Can you work these out from the model? Positions are in its coordinate system, mm. A direction names the side the tool comes from. Coordinates: 2 decimals unless noted, no trailing zeros. Order: outer loops, then holes, each group sorted by start corner. A loop starts at its lowest first (then second) coordinate and runs counter-clockwise, first axis right, second up. Notation, with made-up numbers: (87, 5) -> (140, 5) arc R31 ccw to (140, 31) -> close; hole circle Ø6 at (0.5, 41.25). An arc over 180 degrees is marked (long way). Return JSON: item names as keys, results as strings. Group by question number.
1) Thinking about a two-plate mould opening in Z: for faces 1 (the flat face through (-3, 9, 292.1)), 2 (the flat face through (3, 9, -292.1)), 3 (the flat face through (134, 9, 209.55)), which applies, +Z half, -Z half, draft (parallel to the pull), parting line (faces both ways), or undercut?
2) If we section it at B-B, the plane y = 14: Please give me the cut outline in (x, z), then the cut area to 3 significant figures.
3) For faces 4 (the flat face through (209.55, 9, -112)), 5 (the flat face through (132, 9, 63.5)), 6 (the flat face through (-57.15, 9, 136)), which set-ups out of +Z, -Z, +X, -X, +Y, -Y let a thin tool reach every point of the face, with its end or its side?
4) If I drill on probe 1 along Z at (x, y) = (-160, 1.5); probe 2 along X at (y, z) = (12.25, 132), over which ranges is the centre line in solid material (lowest first)? Write a range as from..to.
5) If we section it at A-A, the plane x = 121: Please give me the cut outline in (y, z).
6) For pin 1 (5.5 mm diameter, centred on y = 9.5, z = 140.5, fed in from -X), with a flat end and sliding along its axis, tell me the tip position at first contact or that it passes through.
Autodesk Inventor part; units mm, degrees
ref_plane "XZ Plane" through (0, 0, 0) normal (0, 1, 0) x (-1, 0, 0)
ref_plane "XY Plane" through (0, 0, 0) normal (0, 0, 1) x (1, 0, 0)
sketch "Sketch1" plane through (0, 0, 0) normal (0, 1, 0) x (-1, 0, 0)
  line L0 (-209.55, 292.1) -> (-209.55, -292.1)
  line L1 (-209.55, -292.1) -> (209.55, -292.1)
  line L2 (209.55, -292.1) -> (209.55, 292.1)
  line L3 (209.55, 292.1) -> (-209.55, 292.1)
  line L4 (-209.55, 292.1) -> (209.55, -292.1) construction
  line L5 (-209.55, -292.1) -> (209.55, 292.1) construction
  point P0 (0, 0)
  dimension "baseLength" = 584.2
  dimension "baseWidth" = 419.1
extrude "Extrusion1" add sketch "Sketch1" along normal blind 17.78
sketch "Sketch2" plane through (0, 0, 0) normal (0, -1, 0) x (1, 0, 0)
  line L0 (209.55, 292.1) -> (209.55, -292.1)
  line L1 (209.55, 209.55) -> (57.15, 209.55)
  line L2 (57.15, 209.55) -> (57.15, 63.5)
  line L3 (57.15, 63.5) -> (209.55, 63.5)
  line L4 (209.55, 63.5) -> (209.55, 209.55)
  line L5 (-209.55, 292.1) -> (209.55, 292.1)
  point P0 (0, 0)
  dimension "backToEndOfGearBox" = 82.55
  dimension "backToFrontOfGearBox" = 228.6
  dimension "wdithForGearBox" = 152.4
extrude "Extrusion2" cut sketch "Sketch2" against normal through all
mirror "Mirror1" about plane through (0, 0, 0) normal (1, 0, 0) of "Extrusion2"
equation "\"baseLength\" = userBaseLength"
equation "\"baseWidth\" = userBaseWidth"
equation "\"spaceingAlongSides\" = 3.175"
equation "\"distanceFromBackForEndBolt\" = 38.1"
equation "\"spacingForBolt\" = 25.4"
equation "\"widthOfSpacingForBolt\" = 12.7"
equation "\"lengthOfSpacingForBolt\" = 25.4"
equation "\"userBaseWidth\" = 419.1"
equation "\"userBaseLength\" = 584.2"
properties part number "RhinoBottomFloorPlate05" material "Wood (Birch)"
Result sheet:
{
 "1": {"face 1": "+Z half", "face 2": "-Z half", "face 3": "undercut"},
 "2": {"outline": "(-209.55, -292.1) -> (209.55, -292.1) -> (209.55, 63.5) -> (57.15, 63.5) -> (57.15, 209.55) -> (209.55, 209.55) -> (209.55, 292.1) -> (-209.55, 292.1) -> (-209.55, 209.55) -> (-57.15, 209.55) -> (-57.15, 63.5) -> (-209.55, 63.5) -> close", "area": "200,000 mm2"},
 "3": {"face 4": "+Z, -Z, +X, +Y, -Y", "face 5": "+X, +Y, -Y", "face 6": "-X, +Y, -Y"},
 "4": {"probe 1": "z = -292.1..63.5, 209.55..292.1", "probe 2": "x = -57.15..57.15"},
 "5": {"outline": "(0, -292.1) -> (17.78, -292.1) -> (17.78, 63.5) -> (0, 63.5) -> close; (0, 209.55) -> (17.78, 209.55) -> (17.78, 292.1) -> (0, 292.1) -> close"},
 "6": {"pin 1": "stops at x = -57.15"}
}
